Model file for the job. Use its own axes, mm. A direction names the side the tool comes from. Coordinates: 2 decimals unless noted, no trailing zeros. Order: outer loops, then holes, each group sorted by start corner. A loop starts at its lowest first (then second) coordinate and runs counter-clockwise, first axis right, second up. Notation, with made-up numbers: (-15.75, -29) -> (-6.75, -29) arc R15 cw to (-6.75, -23) -> close; hole circle Ø5 at (86, -1). An arc over 180 degrees is marked (long way). Use CSV: the item, a comma, the result in double quotes. Start each with the question number.
(1) Cut at A-A on y = -86.5. Write the cut outline in (x, z), plus the area to 3 significant figures.
(2) Pin check, flat tips, straight feed: pin 1 Ø2 at (y, z) = (-224.5, 76.5) entering from -X; pin 2 Ø1 at (y, z) = (-104, -48) entering from -X; pin 3 Ø6 at (x, z) = (123.5, 4) entering from +Y. Stop position of each tip, or through.
(3) Tool access for faces 4 (the cylindrical face through (194.67, -120.25, 3.86)), 5 (the flat face through (53, -280.705, -2)), 6 (the cylindrical face through (-6.104, -4.812, -18.022)), 7 (the flat face through (183, -99, 10)): list every direction of +Z, -Z, +X, -X, +Y, -Y with a clear straight run to the whole face (end or side of a thin tool).
(4) Probe L1, parallel to X at y = -7, z = 0; L2, parallel to X at y = -63, z = -38; L3, parallel to Z at x = 76.5, y = -104. List the from-to ranges inside material, lowest first.
(5) Cut at C-C on y = -196.5. Write the cut outline in (x, z), plus the area to 3 significant figures.
(6) Pull direction Z, two halves, no side cores. Call faces 1 (the flat face through (180, -99, -2.452)), 2 (the flat face through (175.035, -78.401, 3.861)), 3 (the cylindrical face through (92.39, -4.81, 31.64)): pulls with the +Z half, pulls with the -Z half, needs draft (parallel to the pull), parting line crosses it, or undercut.
(7) Cut at B-B on y = -239.5. Write the cut outline in (x, z).
```python
from build123d import *

# Parameters (mm, degrees)
SHELL1_T                 = -8
FILLET1_R                = 12
FILLET3_R                = 20
EXTRUDE_THIN1_DEPTH      = 10
EXTRUDE_THIN1_DEPTH_BACK = 2.451833806


with BuildPart() as part:
    # Sketch2 → Revolve2 (revolve)
    with BuildSketch(Plane.XY):
        with BuildLine():
            Line((-8.874501992, 12.639442231), (-8.874501992, -21.780938926))
            ThreePointArc((-8.874501992, -21.780938926), (-9.786036811, -32.199829586), (-12.492944745, -42.302147526))
            Line((-12.492944745, -42.302147526), (-102.176418507, -288.705466585))
            Line((-102.176418507, -288.705466585), (51.125498008, -288.705466585))
            Line((51.125498008, -288.705466585), (51.125498008, 12.639442231))
            Line((51.125498008, 12.639442231), (-8.874501992, 12.639442231))
        make_face()
    revolve(axis=Axis((51.125498008, 12.639442231, 0), (0, -1, 0)))

    # Shell1
    shell1_openings = [part.faces().sort_by_distance(p)[0] for p in [
        (51.125498008, 12.639442231, 0),
    ]]
    offset(amount=SHELL1_T, openings=shell1_openings, kind=Kind.INTERSECTION)

    # Fillet1
    fillet1_edges = [part.edges().sort_by_distance(p)[0] for p in [
        (193.002230469, -280.705466585, 0),
    ]]
    fillet(fillet1_edges, radius=FILLET1_R)

    # Fillet3
    fillet3_edges = [part.edges().sort_by_distance(p)[0] for p in [
        (204.427414523, -288.705466585, 0),
    ]]
    fillet(fillet3_edges, radius=FILLET3_R)

    # Sketch3 → Extrude-Thin1 (add, two sides)
    with BuildSketch(Plane.XY) as extrude_thin1_sk:
        with BuildLine():
            Line((114.743940761, -42.302147526), (135.417787598, -42.302147526))
            ThreePointArc((135.417787598, -42.302147526), (143.870152833, -44.175991785), (150.73867646, -49.446395332))
            Line((150.73867646, -49.446395332), (200.021007134, -108.178789964))
            ThreePointArc((200.021007134, -108.178789964), (204.624012234, -119.291427303), (202.020626347, -131.034542158))
            Line((202.020626347, -131.034542158), (168.608182886, -188.906591838))
            Line((168.608182886, -188.906591838), (159.947928848, -183.906591838))
            Line((159.947928848, -183.906591838), (193.36037231, -126.034542158))
            ThreePointArc((193.36037231, -126.034542158), (194.662065253, -120.162984731), (192.360562703, -114.606666061))
            Line((192.360562703, -114.606666061), (143.078232029, -55.874271429))
            ThreePointArc((143.078232029, -55.874271429), (139.643970215, -53.239069656), (135.417787598, -52.302147526))
            Line((135.417787598, -52.302147526), (114.743940761, -52.302147526))
            Line((114.743940761, -52.302147526), (114.743940761, -42.302147526))
        make_face()
    extrude(amount=EXTRUDE_THIN1_DEPTH)
    extrude(extrude_thin1_sk.sketch, amount=-EXTRUDE_THIN1_DEPTH_BACK)


solid = part.part
```
Outcome:
1,outline,"circle Ø159.41 at (51.13, 0); (168.78, -2.45) -> (181.83, -2.45) -> (181.83, 10) -> (168.78, 10) -> close; hole circle Ø142.38 at (51.13, 0)"
1,area,"4,200 mm2"
2,pin 1,"x = -54.75"
2,pin 2,"x = -20.72"
2,pin 3,"y = -42.3"
3,face 4,"+Z, -Z"
3,face 5,"none"
3,face 6,"+Y"
3,face 7,"+Z, +X, +Y"
4,L1,"-8.87 to -0.87, 103.13 to 111.13"
4,L2,"-9.03 to 1.33, 100.92 to 111.28"
4,L3,"-82.25 to -73.29, 73.29 to 82.25"
5,outline,"circle Ø239.48 at (51.13, 0); hole circle Ø222.46 at (51.13, 0)"
5,area,"6,180 mm2"
6,face 1,"pulls with the -Z half"
6,face 2,"needs draft"
6,face 3,"undercut"
7,outline,"circle Ø270.79 at (51.13, 0); hole circle Ø253.76 at (51.13, 0)"
